from build123d import *

# Parameters (mm, degrees)
SKETCH_1_R          = 3.75
EXTRUDE_1_DEPTH     = 4
SKETCH_2_R          = 2.5
EXTRUDE_2_DEPTH     = 14
CUT_EXTRUDE_1_DEPTH = 2.5
FILLET_1_R          = 0.1


with BuildPart() as part:
    # 草图1 → 凸台-拉伸1 (new body)
    with BuildSketch(Plane(origin=(0, 0, 0), x_dir=(1, 0, 0), z_dir=(0, 1, 0))):
        with Locations(Location((0, 0, 0), (0, 0, 270))):
            Circle(SKETCH_1_R)
    extrude(amount=EXTRUDE_1_DEPTH)

    # 草图2 → 凸台-拉伸2 (add)
    with BuildSketch(Plane(origin=(0, 4, 0), x_dir=(1, 0, 0), z_dir=(0, 1, 0))):
        with Locations(Location((0, 0, 0), (0, 0, 270))):
            Circle(SKETCH_2_R)
    extrude(amount=EXTRUDE_2_DEPTH)

    # 草图3 → 切除-拉伸1 (cut)
    with BuildSketch(Plane.XZ):
        Polygon((1.241505751, 2.169967667), (-1.258494249, 2.160159352), (-2.5, -0.009808314), (-1.241505751, -2.169967667), (1.258494249, -2.160159352), (2.5, 0.009808314), align=None)
    extrude(amount=-CUT_EXTRUDE_1_DEPTH, mode=Mode.SUBTRACT)

    # 圆角1
    fillet_1_edges = [part.edges().sort_by_distance(p)[0] for p in [
        (1.870752875, 0, 1.089887991),
        (-0.008494249, 0, 2.165063509),
        (-1.879247125, 0, 1.075175519),
        (-1.870752875, 0, -1.089887991),
        (0.008494249, 0, -2.165063509),
        (1.879247125, 0, -1.075175519),
    ]]
    fillet(fillet_1_edges, radius=FILLET_1_R)


solid = part.part
Input: part model. Units: mm. Frame: model coordinates. A direction names the side the tool comes from. Give positions to 0.01 mm unless a question says otherwise; leave off trailing zeros. Write each loop counter-clockwise with the first axis right and the second up, starting at its lowest first coordinate (ties: lowest second). Pieces come first, ordered by that corner, then holes. Notation, with made-up numbers: (-18, -4.75) -> (23, -4.75) arc R12 ccw to (23, 1.25) -> close; hole circle Ø6 at (-8, 25.5). An arc over 180 degrees is marked (long way). Use one line per item in the form item = value. Start each with the question number.
1) Section query A-A on y = 16.5. Return the cut outline in (x, z).
2) Section query B-B on x = -3. Return the cut outline in (y, z), then the cut area to 3 significant figures.
3) Pin query (flat end, axial travel): pin 1 (1 mm diameter, centred on x = 2, y = 14, fed in from -Z); pin 2 (3 mm diameter, centred on y = 12.5, z = -2, fed in from -X); pin 3 (4 mm diameter, centred on x = -2, y = 10, fed in from -Z). Return the tip coordinate at first contact, or that it passes through.
4) Ray query, probe 1 along Y at (x, z) = (1.75, 2); probe 2 along Z at (x, y) = (0.25, 1.25); probe 3 along Y at (x, z) = (-2, -0.25). Return the intervals inside material, ascending. Write a range as from..to.
5) Draft query along X for faces 1 (the cylindrical face through (-2.44, 10.9, -0.54)), 2 (the flat face through (3, 4, 0)), 3 (the flat face through (1.88, 1.283, 1.075)). Return one class per face: pulls with the +X half, pulls with the -X half, needs draft (parallel to the pull), parting line crosses it, or undercut.
6) Set-up query: faces 4 (the flat face through (0, 2.5, 0)), 5 (the flat face through (2, 0, 2)). Return all of +Z, -Z, +X, -X, +Y, -Y with unobstructed straight access to the full face (end or side cutting, diameter ignored); none if empty.
7) Section query C-C on z = 2.75. Return the cut outline in (x, y).
Outcome:
q1.outline = circle Ø5 at (0, 0)
q2.outline = (0, -2.25) -> (4, -2.25) -> (4, 2.25) -> (0, 2.25) -> close
q2.area = 18.0 mm^2
q3.pin_1 = -2
q3.pin_2 = -2.45
q3.pin_3 = -2.5
q4.probe_1 = 0..4
q4.probe_2 = -3.74..-2.16, 2.17..3.74
q4.probe_3 = 2.5..18
q5.face_1 = parting line crosses it
q5.face_2 = needs draft
q5.face_3 = undercut
q6.face_4 = -Y
q6.face_5 = +Z, -Z, +X, -X, -Y
q7.outline = (-2.55, 0) -> (2.55, 0) -> (2.55, 4) -> (-2.55, 4) -> close
